Answer from the drawing. Dimensions are ordinates in mm from the lowest x, y and z of the part. A direction names the side the tool comes from. Coordinates: 2 decimals unless noted, no trailing zeros. Loops run counter-clockwise (first coordinate to the right, second up) from the corner with the lowest first, then second, coordinate; pieces in that order, holes last.
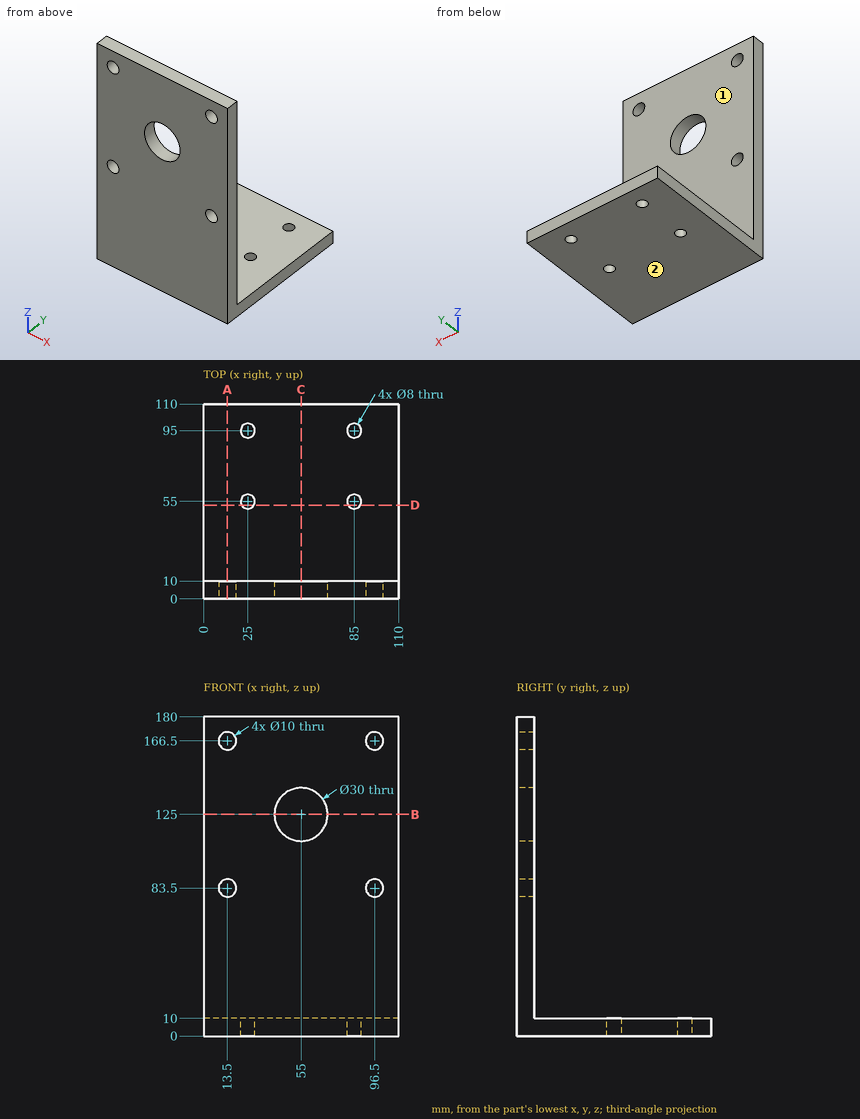
Item 1: Which of the six approach directions +Z, -Z, +X, -X, +Y, -Y give full straight-line access (tool end or side, diameter ignored) to the marked faces 1 and 2?
Numbers:
face 1: +Z, +X, -X, +Y
face 2: -Z, +X, -X, +Y, -Y
Item 2: Find the intervals of material crossed by line 1 along Y through (x, z) = (25, 5.75); line 2 along Z through (x, y) = (55, 7.5); line 3 along X through (y, z) = (55, 2.75), in increasing order.
Numbers:
line 1: y = 0 to 51, 59 to 91, 99 to 110
line 2: z = 0 to 110, 140 to 180
line 3: x = 0 to 21, 29 to 81, 89 to 110
Item 3: A cutting plane is placed at A-A on x = 13.5. Determine the outline of the cut face in (y, z), then the cut area to 3 significant figures.
Numbers:
outline: (0, 0) - (110, 0) - (110, 10) - (10, 10) - (10, 78.5) - (0, 78.5) - close; (0, 88.5) - (10, 88.5) - (10, 161.5) - (0, 161.5) - close; (0, 171.5) - (10, 171.5) - (10, 180) - (0, 180) - close
area: 2,600 mm2
Item 4: A cutting plane is placed at D-D on y = 53. Determine the outline of the cut face in (x, z), then the cut area to 3 significant figures.
Numbers:
outline: (0, 0) - (21.54, 0) - (21.54, 10) - (0, 10) - close; (28.46, 0) - (81.54, 0) - (81.54, 10) - (28.46, 10) - close; (88.46, 0) - (110, 0) - (110, 10) - (88.46, 10) - close
area: 961 mm2
Item 5: Given pin 1 (6 mm diameter, centred on x = 89.5, z = 126.5, fed in from +Y); pin 2 (13 mm diameter, centred on x = 13.5, z = 166.5, fed in from -Y); pin 3 (4 mm diameter, centred on x = 85, y = 28, fed in from +Z); pin 4 (5 mm diameter, centred on x = 85, y = 55, fed in from -Z), each flat-ended and moving along its own axis, determine where each tip first touches the part or whether it passes through.
Numbers:
pin 1: stops at y = 10
pin 2: stops at y = 0
pin 3: stops at z = 10
pin 4: passes through
Item 6: A cutting plane is placed at B-B on z = 125. Determine the outline of the cut face in (x, y), then the cut area to 3 significant figures.
Numbers:
outline: (0, 0) - (40, 0) - (40, 10) - (0, 10) - close; (70, 0) - (110, 0) - (110, 10) - (70, 10) - close
area: 800 mm2
Item 7: A cutting plane is placed at C-C on x = 55. Determine the outline of the cut face in (y, z).
Numbers:
outline: (0, 0) - (110, 0) - (110, 10) - (10, 10) - (10, 110) - (0, 110) - close; (0, 140) - (10, 140) - (10, 180) - (0, 180) - close
